The listing builds one solid part. Answer for the finished solid, in the listing's coordinates (mm). A direction names the side the tool comes from. Coordinates: 2 decimals unless noted, no trailing zeros. Loops run counter-clockwise (first coordinate to the right, second up) from the corner with the lowest first, then second, coordinate; pieces in that order, holes last. Notation, with made-up numbers: (-6.5, 33.25) - (26.5, 33.25) arc R13 cw to (26.5, 58.25) - close; hole circle Ø6 at (24.25, 4.5). An arc over 180 degrees is marked (long way). Put each result on its own line as item: value.
```python
from build123d import *

# Parameters (mm, degrees)
KES_EKSTR_ZYON1_START   = -5
KES_EKSTR_ZYON1_DEPTH   = 5
DAIRESEL_KAPLAMA1_COUNT = 11
RADYUS1_R               = 0.5


with BuildPart() as part:
    # Çizim2 → Döndür1 (revolve)
    with BuildSketch(Plane.XY, mode=Mode.PRIVATE) as d_nd_r1_sk:
        Polygon((0, 0), (0, 26.1), (1, 26.1), (1, 26), (2, 26), (2, 22), (1, 22), (1, 18.541448382), (4, 18.541448382), (4, 0), align=None)
    revolve(d_nd_r1_sk.sketch.rotate(Axis((0, 0, 0), (0, 1, 0)), 90), axis=Axis((0, 0, 0), (0, 1, 0)))

    # Çizim4 → Kes-Ekstrüzyon1 (cut)
    with BuildSketch(Plane(origin=(0, 26, 0), x_dir=(1, 0, 0), z_dir=(0, 1, 0)).offset(KES_EKSTR_ZYON1_START)):
        with BuildLine():
            ThreePointArc((-0.5, 1.936491673), (0, 2), (0.5, 1.936491673))
            ThreePointArc((0.5, 1.936491673), (0.260400333, 1.599188187), (0.095331419, 1.219801979))
            ThreePointArc((0.095331419, 1.219801979), (0, 1.15), (-0.095331419, 1.219801979))
            ThreePointArc((-0.095331419, 1.219801979), (-0.260400333, 1.599188187), (-0.5, 1.936491673))
        make_face()
    kes_ekstr_zyon1 = extrude(amount=KES_EKSTR_ZYON1_DEPTH, mode=Mode.SUBTRACT)

    # Dairesel Kaplama1: Kes-Ekstrüzyon1 ×11 about axis
    dairesel_kaplama1_axis = Axis((0, 0, 0), (0, 1, 0))
    for i in range(1, DAIRESEL_KAPLAMA1_COUNT):
        add(kes_ekstr_zyon1.rotate(dairesel_kaplama1_axis, i * 360 / DAIRESEL_KAPLAMA1_COUNT), mode=Mode.SUBTRACT)

    # Radyus1
    radyus1_edges = [part.edges().sort_by_distance(p)[0] for p in [
        (0, 18.541448382, 4),
    ]]
    fillet(radyus1_edges, radius=RADYUS1_R)


solid = part.part
```
1) For a pull along Y with two mould halves and no side action, classify faces 1 (the face through (0, 0, 0)), 2 (the face through (1, 20, 0)), 3 (the face through (0.645, 23.972, -1.48)), 4 (the face through (0, 26.1, 0)) as pulls with the +Y half, pulls with the -Y half, needs draft (parallel to the pull), parting line crosses it, or undercut.
Found:
face 1: pulls with the -Y half
face 2: undercut
face 3: needs draft
face 4: pulls with the +Y half
2) Straight lines are drawn through the part: L1, parallel to Y at x = 1, z = -0.25; L2, parallel to Y at x = 1.5, z = 1; L3, parallel to Z at x = 3.5, y = 1.5. For each, find the intervals that lie inside material, in ascending order. Write a range as [from, to].
Found:
L1: y = [0, 18.54], [22, 26]
L2: y = [0, 18.54]
L3: z = [-1.94, 1.94]
3) The part is cut by section A-A (y = 16.25). Give the vertices of the cut face in (x, z), and give its area (3 significant figures).
Found:
outline: circle Ø8 at (0, 0)
area: 50.3 mm^2
4) For faces 5 (the face through (1, 18.541, 1)), 6 (the face through (3.905, 8.894, 0.867)), 7 (the face through (-0.202, 23.972, 1.602)), 8 (the face through (1.37, 23.97, 0.85)), determine the directions among +Z, -Z, +X, -X, +Y, -Y from which every point of the face is accessible in a straight line to the end or side of a thin tool.
Found:
face 5: none
face 6: +Y, -Y
face 7: +Z, +Y
face 8: +Y
